Could you check a few things on this model? Use its own coordinates, in mm. A direction names the side the tool comes from. Round coordinates to 2 decimals unless told otherwise and drop trailing zeros. Loops run counter-clockwise (first coordinate to the right, second up) from the corner with the lowest first, then second, coordinate; pieces in that order, holes last. Notation, with made-up numbers: M -27,26.25 L -6,26.25 A17 cw -6,44.25 Z; hole C 65.5,5.25 d7. An arc over 180 degrees is marked long. One line per item, written item: value. Start each with the question number.
Q1. I'm going to push flat-ended pins straight in: pin 1 Ø4 at (x, y) = (-6, 41.5) entering from -Z; pin 2 Ø6 at (y, z) = (51, -5.5) entering from +X; pin 3 Ø10 at (x, y) = (-6.5, 31) entering from -Z. Where does each tip first touch, or does it pass through?
Q2. Imagine slicing it at C-C (y = 31). Please give me the cut outline in (x, z).
Q3. Please list where these lines run through material, in increasing order: line 1 along X through (y, z) = (64.4, 0); line 2 along Y through (x, z) = (3.5, -3.25); line 3 along Z through (x, y) = (0.25, 10).
Q4. Which directions (+Z, -Z, +X, -X, +Y, -Y) give clear straight access to the entire face, cutting with the end or side of a thin tool? Please do faces 4 (the face through (0, 0, 0)), 5 (the face through (1.352, 64.707, 4.292)).
Q5. Imagine slicing it at D-D (x = 5.75). Please give me the cut outline in (y, z), then the cut area to 3 significant figures.
Q6. Imagine slicing it at A-A (x = -3). Please give me the cut outline in (y, z).
Q7. Imagine slicing it at B-B (z = -2.75). Please give me the cut outline in (x, y).
Q8. Thinking about a two-plate mould opening in X: for faces 1 (the face through (2.914, 32.144, 9.252)), 2 (the face through (7, 65.2, -3)), 3 (the face through (-6.834, 64.707, -1.517)), which applies, released by +X, released by -X, zero draft, split by the parting line, or undercut?
from build123d import *

# Parameters (mm, degrees)
SKETCH2_R           = 9.7
BOSS_EXTRUDE1_DEPTH = 65.2
SKETCH3_R           = 7
SKETCH3_R_2         = 4.5
CUT_EXTRUDE1_DEPTH  = 1


with BuildPart() as part:
    # Sketch2 → Boss-Extrude1 (new body)
    with BuildSketch(Plane(origin=(0, 0, 0), x_dir=(1, 0, 0), z_dir=(0, 1, 0))):
        with Locations(Location((0, 0, 0), (0, 0, 270))):
            Circle(SKETCH2_R)
    extrude(amount=BOSS_EXTRUDE1_DEPTH)

    # Sketch3 → Cut-Extrude1 (cut)
    with BuildSketch(Plane(origin=(0, 65.2, 0), x_dir=(1, 0, 0), z_dir=(0, 1, 0))):
        with Locations(Location((0, 0, 0), (0, 0, 270))):
            Circle(SKETCH3_R)
        with Locations(Location((0, 0, 0), (0, 0, 270))):
            Circle(SKETCH3_R_2, mode=Mode.SUBTRACT)
    extrude(amount=-CUT_EXTRUDE1_DEPTH, mode=Mode.SUBTRACT)


solid = part.part
Report:
1. pin 1: stops at z = -8.84
1. pin 2: stops at x = 9.37
1. pin 3: stops at z = -9.58
2. outline: C 0,0 d19.4
3. line 1: x = -9.7 to -7, -4.5 to 4.5, 7 to 9.7
3. line 2: y = 0 to 64.2
3. line 3: z = -9.7 to 9.7
4. face 4: +Z, -Z, +X, -X, -Y
4. face 5: +Y
5. outline: M 0,-7.81 L 65.2,-7.81 L 65.2,-3.99 L 64.2,-3.99 L 64.2,3.99 L 65.2,3.99 L 65.2,7.81 L 0,7.81 Z
5. area: 1,010 mm²
6. outline: M 0,-9.22 L 65.2,-9.22 L 65.2,-6.32 L 64.2,-6.32 L 64.2,-3.35 L 65.2,-3.35 L 65.2,3.35 L 64.2,3.35 L 64.2,6.32 L 65.2,6.32 L 65.2,9.22 L 0,9.22 Z
7. outline: M -9.3,0 L 9.3,0 L 9.3,65.2 L 6.44,65.2 L 6.44,64.2 L 3.56,64.2 L 3.56,65.2 L -3.56,65.2 L -3.56,64.2 L -6.44,64.2 L -6.44,65.2 L -9.3,65.2 Z
8. face 1: split by the parting line
8. face 2: zero draft
8. face 3: undercut
